Check sheet for the modelled part. Datum: model origin and axes. Units: mm. Round coordinates to 2 decimals unless told otherwise and drop trailing zeros. Loops run counter-clockwise (first coordinate to the right, second up) from the corner with the lowest first, then second, coordinate; pieces in that order, holes last. Notation, with made-up numbers: (-24, 67) -> (27, 67) arc R19 ccw to (27, 78) -> close; hole circle Ø9 at (29, 48.25). An arc over 180 degrees is marked (long way). One line per item, written item: value. Start each with the question number.
1. Cross-section at A-A on y = 45.72. Record the cut outline in (x, z) (3 decimals).
2. Cross-section at D-D on z = -1.15. Count the separate pieces of the cut face and the enclosed holes in it, then the cut area to 3 significant figures.
3. Cross-section at C-C on x = -31.75. Record the cut outline in (y, z) (3 decimals).
4. Material ranges on L1, parallel to X at y = 69.5, z = -0.8; L2, parallel to Y at x = -72, z = -0.15; L3, parallel to Y at x = -29.5, z = -0.55, recorded low to high.
5. Go/stop test with a flat-tipped pin: pin 1 (2.5 mm diameter, centred on x = -31.75, y = 69.7, fed in from -Z). Record where the tip stops, or that it passes through.
6. Cross-section at B-B on x = -72.39. Record the cut outline in (y, z) (3 decimals), then the cut area to 3 significant figures.
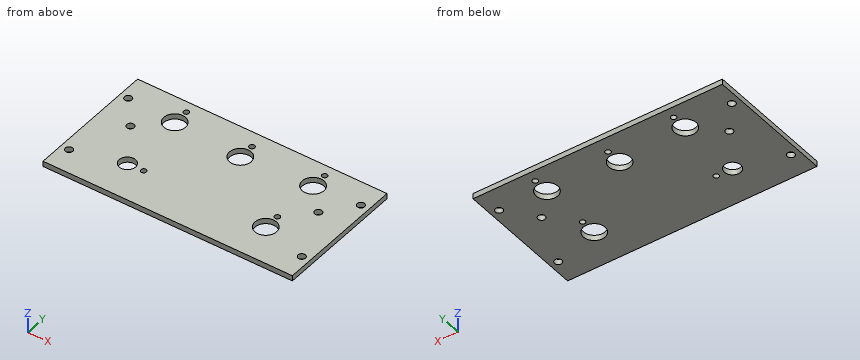
from build123d import *

# Parameters (mm, degrees)
SKETCH1_W                    = 146.05
SKETCH1_H                    = 76.2
BOSS_EXTRUDE1_DEPTH          = 3.175
F_6_CLEARANCE_HOLE1_D        = 4.3053
F_3_8_0_375_DIAMETER_HOLE1_D = 9.525
F_1_2_0_5_DIAMETER_HOLE1_D   = 12.7
F_1_8_0_125_DIAMETER_HOLE1_D = 3.175


with BuildPart() as part:
    # Sketch1 → Boss-Extrude1 (new body)
    with BuildSketch(Plane.XY):
        with Locations((-73.025, 38.1)):
            Rectangle(SKETCH1_W, SKETCH1_H)
    extrude(amount=-BOSS_EXTRUDE1_DEPTH)

    # #6 Clearance Hole1 (through all)
    with Locations(Plane(origin=(0, 0, -3.175), x_dir=(-1, 0, 0), z_dir=(0, 0, -1))):
        with Locations((4.8895, 61.9125), (4.8895, 14.2875), (141.1605, 14.2875), (141.1605, 61.9125), (128.016, 45.72), (18.034, 45.72)):
            Hole(F_6_CLEARANCE_HOLE1_D / 2)

    # 3/8 (0.375) Diameter Hole1 (through all)
    with Locations(Plane(origin=(0, 0, -3.175), x_dir=(-1, 0, 0), z_dir=(0, 0, -1))):
        with Locations((112.776, 22.225)):
            Hole(F_3_8_0_375_DIAMETER_HOLE1_D / 2)

    # 1/2 (0.5) Diameter Hole1 (through all)
    with Locations(Plane(origin=(0, 0, -3.175), x_dir=(-1, 0, 0), z_dir=(0, 0, -1))):
        with Locations((31.75, 60.325), (72.39, 57.658), (112.776, 60.325), (31.75, 22.225)):
            Hole(F_1_2_0_5_DIAMETER_HOLE1_D / 2)

    # 1/8 (0.125) Diameter Hole1 (through all)
    with Locations(Plane(origin=(0, 0, -3.175), x_dir=(-1, 0, 0), z_dir=(0, 0, -1))):
        with Locations((31.75, 69.699492067), (112.776, 69.699492067), (103.251, 22.225), (72.39, 67.032492067), (31.75, 31.599492067)):
            Hole(F_1_8_0_125_DIAMETER_HOLE1_D / 2)


solid = part.part
Taken from the geometry:
1. outline: (-146.05, -3.175) -> (-130.169, -3.175) -> (-130.169, 0) -> (-146.05, 0) -> close; (-125.863, -3.175) -> (-20.187, -3.175) -> (-20.187, 0) -> (-125.863, 0) -> close; (-15.881, -3.175) -> (0, -3.175) -> (0, 0) -> (-15.881, 0) -> close
2. separate pieces: 1
2. enclosed holes: 16
2. area: 10,400 mm2
3. outline: (0, -3.175) -> (15.875, -3.175) -> (15.875, 0) -> (0, 0) -> close; (28.575, -3.175) -> (30.012, -3.175) -> (30.012, 0) -> (28.575, 0) -> close; (33.187, -3.175) -> (53.975, -3.175) -> (53.975, 0) -> (33.187, 0) -> close; (66.675, -3.175) -> (68.112, -3.175) -> (68.112, 0) -> (66.675, 0) -> close; (71.287, -3.175) -> (76.2, -3.175) -> (76.2, 0) -> (71.287, 0) -> close
4. L1: x = -146.05 to -114.35, -111.2 to -33.32, -30.18 to 0
4. L2: y = 0 to 51.32, 64 to 65.49, 68.57 to 76.2
4. L3: y = 0 to 16.29, 28.16 to 54.39, 66.26 to 76.2
5. pin 1: passes through
6. outline: (0, -3.175) -> (51.308, -3.175) -> (51.308, 0) -> (0, 0) -> close; (64.008, -3.175) -> (65.445, -3.175) -> (65.445, 0) -> (64.008, 0) -> close; (68.62, -3.175) -> (76.2, -3.175) -> (76.2, 0) -> (68.62, 0) -> close
6. area: 192 mm2
